from build123d import *

# Parameters (mm, degrees)
F1_DEPTH      = 25
F1_TAPER      = -3
F1_DEPTH_BACK = 25


with BuildPart() as f1:
    # F0 (on Front) → F1 (new body, two sides)
    with BuildSketch(Plane.XZ) as f1_sk:
        Polygon((0, 60), (0, 0), (40, 0), (40, 10), (12, 10), (12, 35), (6, 35), (6, 60), align=None)
    extrude(amount=F1_DEPTH, taper=F1_TAPER)
    extrude(f1_sk.sketch, amount=-F1_DEPTH_BACK)


solid = f1.part
Model file for the job. Use its own axes, mm. A direction names the side the tool comes from. Coordinates: 2 decimals unless noted, no trailing zeros. Loops run counter-clockwise (first coordinate to the right, second up) from the corner with the lowest first, then second, coordinate; pieces in that order, holes last. Notation, with made-up numbers: (50.5, -15.75) -> (103.5, -15.75) arc R21 cw to (103.5, 16.25) -> close; hole circle Ø8 at (-10, 40). An arc over 180 degrees is marked (long way). Use one line per item in the form item = value. Start each with the question number.
(1) Cut at A-A on y = 2.5. Give the cut face in (x, z).
(2) Flat gauge pins, fed straight in: pin 1 (6 mm diameter, centred on x = 13.5, y = -1, fed in from -Z); pin 2 (8 mm diameter, centred on y = -14, z = 30.5, fed in from -X); pin 3 (6.5 mm diameter, centred on x = 3.5, y = 9, fed in from +Z). Where does each tip first touch, or does it go through?
(3) Tool access for faces 1 (the flat face through (20, 12, 0)), 2 (the flat face through (40, 12, 5)), 3 (the flat face through (0, 12, 30)), 4 (the flat face through (9, 12, 35)), 5 (the flat face through (3, 12, 60)): list every direction of +Z, -Z, +X, -X, +Y, -Y with a clear straight run to the whole face (end or side of a thin tool).
(4) Probe probe 1 along Z at (x, y) = (2, 11); probe 2 along X at (y, z) = (8, 20.5); probe 3 along X at (y, z) = (18, 48). List the from-to ranges inside material, lowest first. Write a range as from..to.
Values:
q1.outline = (0, 0) -> (40, 0) -> (40, 10) -> (12, 10) -> (12, 35) -> (6, 35) -> (6, 60) -> (0, 60) -> close
q2.pin_1 = -0.21
q2.pin_2 = -0.94
q2.pin_3 = 60
q3.face_1 = -Z, +X, -X, +Y
q3.face_2 = +Z, -Z, +X, +Y
q3.face_3 = +Z, -Z, -X, +Y
q3.face_4 = +Z, +X, +Y
q3.face_5 = +Z, +X, -X, +Y
q4.probe_1 = 0..60
q4.probe_2 = 0..12
q4.probe_3 = 0..6
